Model file for the job. Use its own axes, mm. A direction names the side the tool comes from. Give positions to 0.01 mm unless a question says otherwise; leave off trailing zeros. Loops run counter-clockwise (first coordinate to the right, second up) from the corner with the lowest first, then second, coordinate; pieces in that order, holes last. Notation, with made-up numbers: (-27.5, -4) - (11.5, -4) arc R8 cw to (11.5, 8) - close; hole circle Ø1 at (35.5, 66). An arc over 180 degrees is marked (long way). Answer as CSV lines item,"result". Start each with the question number.
Item 1: Tool access for faces 4 (the flat face through (26, 3, -1)), 5 (the flat face through (1.2, 4, -38)), 6 (the flat face through (2.6, 5.3, -31.4)), 7 (the flat face through (38.5, 1.2, -27.9)): list every direction of +Z, -Z, +X, -X, +Y, -Y with a clear straight run to the whole face (end or side of a thin tool).
Item 2: Drill centre lines: L1, parallel to X at y = 5.25, z = -4; L2, parallel to Z at x = 4, y = 4.75; L3, parallel to X at y = 3.1, z = -30.5. Where is each one in solid material? Low to high. Write a range as from..to.
Item 3: Pin check, flat tips, straight feed: pin 1 (0.9 mm diameter, centred on x = 28, y = 2.5, fed in from -Z); pin 2 (4 mm diameter, centred on y = 3, z = -31.5, fed in from -X); pin 3 (1.3 mm diameter, centred on y = 4, z = -43.5, fed in from -X); pin 4 (1 mm diameter, centred on x = 43.5, y = 3, fed in from -Z). Stop position of each tip, or through.
Item 4: Pull direction Z, two halves, no side cores. Call faces 1 (the flat face through (27.5, 1.2, -3.4)), 2 (the flat face through (22, 0, -8)), 3 (the flat face through (27, 3, -9)): pulls with the +Z half, pulls with the -Z half, needs draft (parallel to the pull), parting line crosses it, or undercut.
Item 5: Saw through at A-A on x = 13.5. Give the cut face in (y, z).
Item 6: Saw through at C-C on z = -33. Give the cut face in (x, y).
Item 7: Saw through at B-B on y = 3.5. State how many separate pieces and enclosed holes the cut face has, plus the area to 3 significant figures.
from build123d import *

# Parameters (mm, degrees)
SKETCH1_R           = 1.5
BOSS_EXTRUDE1_DEPTH = 1.2
BOSS_EXTRUDE4_DEPTH = 6
SKETCH5_W           = 6
SKETCH5_H           = 8
BOSS_EXTRUDE8_DEPTH = 4.1
SKETCH1_3_R         = 1.5
CUT_EXTRUDE1_DEPTH  = 2.5
SKETCH1_4_R         = 1.5
CUT_EXTRUDE2_DEPTH  = 63.640561939


with BuildPart() as part:
    # Sketch1 → Boss-Extrude1 (new body)
    with BuildSketch(Plane(origin=(0, 0, 0), x_dir=(1, 0, 0), z_dir=(0, 1, 0))):
        with BuildLine():
            Line((3, 0), (41, 0))
            ThreePointArc((41, 0), (43.121320344, 0.878679656), (44, 3))
            Line((44, 3), (44, 41))
            ThreePointArc((44, 41), (43.121320344, 43.121320344), (41, 44))
            Line((41, 44), (3, 44))
            ThreePointArc((3, 44), (0.878679656, 43.121320344), (0, 41))
            Line((0, 41), (0, 3))
            ThreePointArc((0, 3), (0.878679656, 0.878679656), (3, 0))
        make_face()
        with Locations(Location((4, 30.5, 0), (0, 0, 270))):
            Circle(SKETCH1_R, mode=Mode.SUBTRACT)
        with Locations(Location((40, 30.5, 0), (0, 0, 270))):
            Circle(SKETCH1_R, mode=Mode.SUBTRACT)
        with Locations(Location((26, 6, 0), (0, 0, 270))):
            Circle(SKETCH1_R, mode=Mode.SUBTRACT)
        with BuildLine():
            Line((31.656854249, 8), (36, 8))
            Line((36, 8), (36, 40))
            Line((36, 40), (8, 40))
            Line((8, 40), (8, 8))
            Line((8, 8), (20.343145751, 8))
            ThreePointArc((20.343145751, 8), (26, 12), (31.656854249, 8))
        make_face(mode=Mode.SUBTRACT)
    extrude(amount=BOSS_EXTRUDE1_DEPTH)

    # Sketch4 → Boss-Extrude4 (add)
    with BuildSketch(Plane(origin=(0, 1.2, 0), x_dir=(1, 0, 0), z_dir=(0, 1, 0))):
        with BuildLine():
            Line((8, 44), (3, 44))
            ThreePointArc((3, 44), (0.878679656, 43.121320344), (0, 41))
            Line((0, 41), (0, 36))
            Line((0, 36), (1.2, 36))
            Line((1.2, 36), (1.2, 41))
            ThreePointArc((1.2, 41), (1.727207794, 42.272792206), (3, 42.8))
            Line((3, 42.8), (8, 42.8))
            Line((8, 42.8), (8, 44))
        make_face()
        with BuildLine():
            ThreePointArc((44, 41), (43.121320344, 43.121320344), (41, 44))
            Line((41, 44), (36, 44))
            Line((36, 44), (36, 42.8))
            Line((36, 42.8), (41, 42.8))
            ThreePointArc((41, 42.8), (42.272792206, 42.272792206), (42.8, 41))
            Line((42.8, 41), (42.8, 36))
            Line((42.8, 36), (44, 36))
            Line((44, 36), (44, 41))
        make_face()
        with BuildLine():
            Line((36, 0), (41, 0))
            ThreePointArc((41, 0), (43.121320344, 0.878679656), (44, 3))
            Line((44, 3), (44, 8))
            Line((44, 8), (42.8, 8))
            Line((42.8, 8), (42.8, 3))
            ThreePointArc((42.8, 3), (42.272792206, 1.727207794), (41, 1.2))
            Line((41, 1.2), (36, 1.2))
            Line((36, 1.2), (36, 0))
        make_face()
        with BuildLine():
            ThreePointArc((0, 3), (0.878679656, 0.878679656), (3, 0))
            Line((3, 0), (8, 0))
            Line((8, 0), (8, 1.2))
            Line((8, 1.2), (3, 1.2))
            ThreePointArc((3, 1.2), (1.727207794, 1.727207794), (1.2, 3))
            Line((1.2, 3), (1.2, 8))
            Line((1.2, 8), (0, 8))
            Line((0, 8), (0, 3))
        make_face()
    extrude(amount=BOSS_EXTRUDE4_DEPTH)

    # Sketch5 → Boss-Extrude8 (add)
    with BuildSketch(Plane(origin=(0, 1.2, 0), x_dir=(1, 0, 0), z_dir=(0, 1, 0))):
        with Locations((4, 30.5)):
            Rectangle(SKETCH5_W, SKETCH5_H)
        with Locations((40, 30.5)):
            Rectangle(SKETCH5_W, SKETCH5_H)
        with BuildLine():
            Line((26, 9), (29, 9))
            Line((29, 9), (29, 1))
            Line((29, 1), (23, 1))
            Line((23, 1), (23, 6))
            ThreePointArc((23, 6), (23.878679656, 8.121320344), (26, 9))
        make_face()
    extrude(amount=BOSS_EXTRUDE8_DEPTH)

    # Sketch1_3 → Cut-Extrude1 (cut)
    # profile 1 of 3: a face of its own
    with BuildSketch(Plane(origin=(0, 0, 0), x_dir=(1, 0, 0), z_dir=(0, 1, 0))):
        Polygon((7, 32.232050808), (4, 33.964101615), (1, 32.232050808), (1, 28.767949192), (4, 27.035898385), (7, 28.767949192), align=None)
        with Locations(Location((4, 30.5, 0), (0, 0, 270))):
            Circle(SKETCH1_3_R, mode=Mode.SUBTRACT)
    # profile 2 of 3: a face of its own
    with BuildSketch(Plane(origin=(0, 0, 0), x_dir=(1, 0, 0), z_dir=(0, 1, 0))):
        Polygon((29, 7.732050808), (26, 9.464101615), (23, 7.732050808), (23, 4.267949192), (26, 2.535898385), (29, 4.267949192), align=None)
        with Locations(Location((26, 6, 0), (0, 0, 270))):
            Circle(SKETCH1_3_R, mode=Mode.SUBTRACT)
    # profile 3 of 3: a face of its own
    with BuildSketch(Plane(origin=(0, 0, 0), x_dir=(1, 0, 0), z_dir=(0, 1, 0))):
        Polygon((43, 32.232050808), (40, 33.964101615), (37, 32.232050808), (37, 28.767949192), (40, 27.035898385), (43, 28.767949192), align=None)
        with Locations(Location((40, 30.5, 0), (0, 0, 270))):
            Circle(SKETCH1_3_R, mode=Mode.SUBTRACT)
    extrude(amount=CUT_EXTRUDE1_DEPTH, mode=Mode.SUBTRACT)

    # Sketch1_4 → Cut-Extrude2 (cut, through all)
    with BuildSketch(Plane(origin=(0, 0, 0), x_dir=(1, 0, 0), z_dir=(0, 1, 0))):
        with Locations(Location((4, 30.5, 0), (0, 0, 270))):
            Circle(SKETCH1_4_R)
        with Locations(Location((26, 6, 0), (0, 0, 270))):
            Circle(SKETCH1_4_R)
        with Locations(Location((40, 30.5, 0), (0, 0, 270))):
            Circle(SKETCH1_4_R)
    extrude(amount=CUT_EXTRUDE2_DEPTH, mode=Mode.SUBTRACT)


solid = part.part
Responses:
1,face 4,"+Z, +Y"
1,face 5,"+Y"
1,face 6,"+X, -X, +Y"
1,face 7,"-Y"
2,L1,"0..1.2, 23..29, 42.8..44"
2,L2,"-44..-42.8, -34.5..-32, -29..-26.5, -1.2..0"
2,L3,"1..2.5, 5.5..7, 37..38.5, 41.5..43"
3,pin 1,"z = -9"
3,pin 2,"x = 0"
3,pin 3,"x = 0.64"
3,pin 4,"z = -43.24"
4,face 1,"undercut"
4,face 2,"needs draft"
4,face 3,"pulls with the -Z half"
5,outline,"(0, -44) - (1.2, -44) - (1.2, -40) - (0, -40) - close; (0, -8) - (1.2, -8) - (1.2, 0) - (0, 0) - close"
6,outline,"(0, 0) - (2.33, 0) - (2.33, 2.5) - (5.67, 2.5) - (5.67, 0) - (8, 0) - (8, 1.2) - (7, 1.2) - (7, 5.3) - (1, 5.3) - (1, 1.2) - (0, 1.2) - close; (36, 0) - (38.33, 0) - (38.33, 2.5) - (41.67, 2.5) - (41.67, 0) - (44, 0) - (44, 1.2) - (43, 1.2) - (43, 5.3) - (37, 5.3) - (37, 1.2) - (36, 1.2) - close"
7,separate pieces,"7"
7,enclosed holes,"3"
7,area,"187 mm2"
